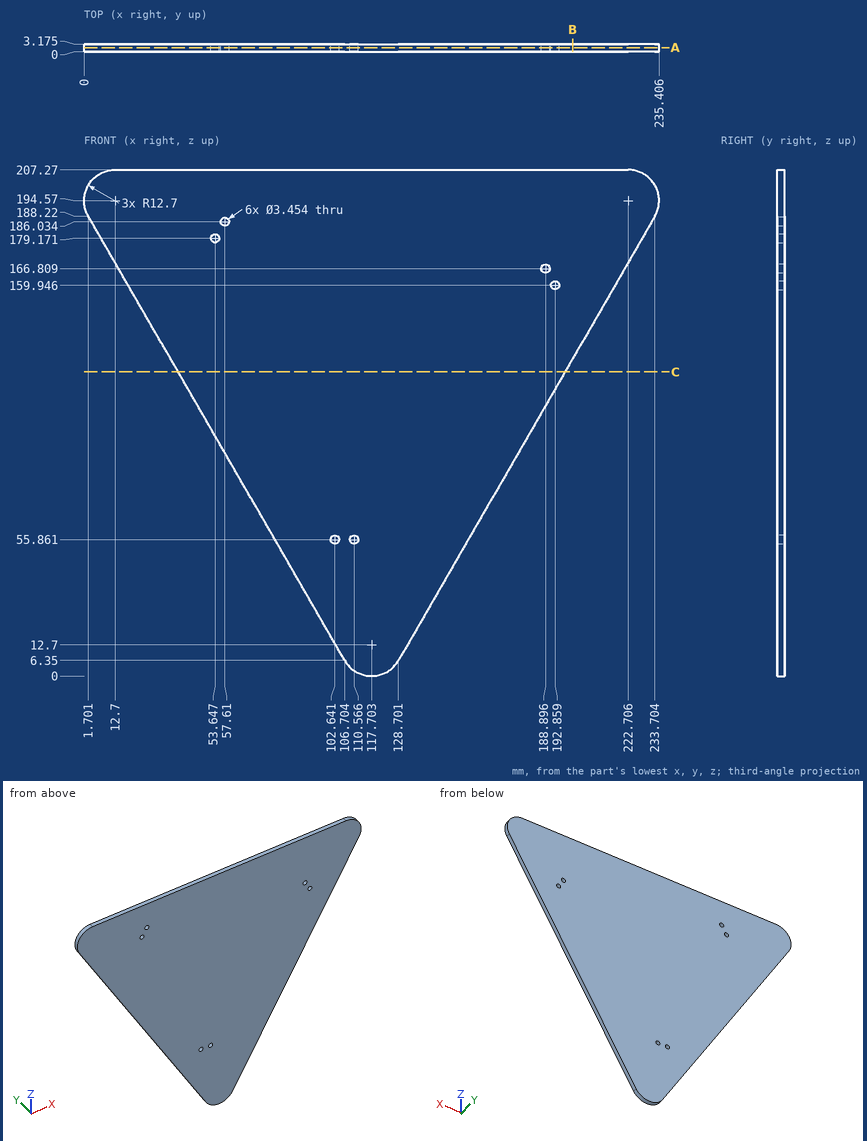
Geometry check sheet. Reference: drawing and pictorial views, mm from the part's lowest x, y, z. Coordinates: 2 decimals unless noted, no trailing zeros. Loops run counter-clockwise (first coordinate to the right, second up) from the corner with the lowest first, then second, coordinate; pieces in that order, holes last.
1) Sectioned sample at A-A (y = 1.7). Count the separate pieces of the cut face and the enclosed holes in it, and give its area (3 significant figures).
2) Sectioned sample at C-C (z = 124.5). Record the boundary of the cut face in (x, y) (1 decimal), and give its area (3 significant figures).
3) Material ranges on probe 1 along Z at (x, y) = (189.5, 2.65) (1 decimal); probe 2 along X at (y, z) = (0.9, 159) (1 decimal); probe 3 along Z at (x, y) = (70.5, 2.85) (1 decimal), recorded low to high.
4) Sectioned sample at B-B (x = 200). Record the boundary of the cut face in (y, z) (1 decimal).
Check sheet entries:
1. separate pieces: 1
1. enclosed holes: 6
1. area: 27,500 mm2
2. outline: (38.5, 0) - (196.9, 0) - (196.9, 3.2) - (38.5, 3.2) - close
2. area: 503 mm2
3. probe 1: z = 111.7 to 165.2, 168.4 to 207.3
3. probe 2: x = 18.6 to 191.4, 194.3 to 216.8
3. probe 3: z = 69.1 to 207.3
4. outline: (0, 129.8) - (3.2, 129.8) - (3.2, 207.3) - (0, 207.3) - close
